Solid Edge part; units mm, degrees
sketch "Sketch1" plane through (0, 0, 0) normal (0, 0, 1) x (1, 0, 0)
  circle A0 centre (34.5, 34.5) radius 1.65
  circle A1 centre (-34.5, 34.5) radius 1.65
  circle A2 centre (-34.5, -34.5) radius 1.65
  circle A3 centre (34.5, -34.5) radius 1.65
  line L0 (42.5, 42.5) -> (-42.5, 42.5)
  line L1 (-42.5, 42.5) -> (-42.5, -42.5)
  line L2 (-42.5, -42.5) -> (42.5, -42.5)
  line L3 (42.5, -42.5) -> (42.5, 42.5)
extrude "Protrusion1" add sketch "Sketch1" against normal blind 3.5
sketch "Sketch2" plane through (0, 0, 0) normal (0, 0, 1) x (1, 0, 0)
  circle A0 centre (0, 0) radius 31
  circle A1 centre (0, 0) radius 37.9
extrude "ExtrudedProtrusion_2" add sketch "Sketch2" along normal blind 6.5
chamfer "Chamfer_1" distance 0.5 angle 45 1 edges at (-37.9, 0, 6.5)
chamfer "Chamfer_2" distance 1.8 angle 45 1 edges at (-31, 0, 0)
Can you work these out from the model? Positions are in its coordinate system, mm. A direction names the side the tool comes from. Coordinates: 2 decimals unless noted, no trailing zeros. Loops run counter-clockwise (first coordinate to the right, second up) from the corner with the lowest first, then second, coordinate; pieces in that order, holes last. Notation, with made-up numbers: (19, 17.25) - (38, 17.25) arc R30 ccw to (38, 41.25) - close; hole circle Ø1 at (85.5, 63). An arc over 180 degrees is marked (long way). Put each result on its own line as item: value. Start each with the question number.
Item 1: Suppose I cut it at B-B (x = 34.5). State how many separate pieces and enclosed holes the cut face has, and give its area (3 significant figures).
Item 2: For pin 1 (2 mm diameter, centred on x = -21, y = 4, fed in from +Z); pin 2 (1 mm diameter, centred on x = 31.5, z = 4, fed in from -Y), each with a flat end and sliding along its axis, tell me the tip position at first contact or that it passes through.
Item 3: Suppose I cut it at A-A (y = 0). Please give me the cut outline in (x, z).
Item 4: Which directions (+Z, -Z, +X, -X, +Y, -Y) give clear straight access to the entire face, cutting with the end or side of a thin tool? Please do faces 1 (the face through (-1, -42.5, -2)), 2 (the face through (0, 0, 0)).
Item 5: If I drill on line 1 along Y through (x, z) = (-34.5, -0.8); line 2 along Z through (x, y) = (-6.5, 19); line 3 along X through (y, z) = (14.5, 0.25), over which ranges is the centre line in solid material (lowest first)?
Item 6: If we mould it in two halves opening along X, with no side actions, what happens to faces 3 (the face through (33.284, -33.385, -1.726)), 4 (the face through (-42.5, 1, -2)), 5 (the face through (1, 42.5, -2))? For each: +X half, -X half, draft (parallel to the pull), parting line (faces both ways), or undercut.
Here are the results:
1. separate pieces: 3
1. enclosed holes: 0
1. area: 478 mm²
2. pin 1: z = 0
2. pin 2: y = -21.8
3. outline: (-42.5, -3.5) - (42.5, -3.5) - (42.5, 0) - (37.9, 0) - (37.9, 6) - (37.4, 6.5) - (31, 6.5) - (31, 1.8) - (29.2, 0) - (-29.2, 0) - (-31, 1.8) - (-31, 6.5) - (-37.4, 6.5) - (-37.9, 6) - (-37.9, 0) - (-42.5, 0) - close
4. face 1: +Z, -Z, +X, -X, -Y
4. face 2: +Z
5. line 1: -42.5 to -36.15, -32.85 to 32.85, 36.15 to 42.5
5. line 2: -3.5 to 0
5. line 3: -35.02 to -25.63, 25.63 to 35.02
6. face 3: undercut
6. face 4: -X half
6. face 5: draft
